from build123d import *

# Parameters (mm, degrees)
SKETCH1_W           = 601
SKETCH1_H           = 1100
SKETCH1_R           = 200
BOSS_EXTRUDE1_DEPTH = 1900
SKETCH2_W           = 1900
SKETCH2_H           = 340
CUT_EXTRUDE1_DEPTH  = 300
SKETCH3_R           = 15
SKETCH3_R_2         = 50
CUT_EXTRUDE2_DEPTH  = 2277.225164609


with BuildPart() as part:
    # Sketch1 → Boss-Extrude1 (new body)
    with BuildSketch(Plane(origin=(0, 0, 0), x_dir=(0, 0, -1), z_dir=(1, 0, 0))):
        with Locations((300.5, 550)):
            Rectangle(SKETCH1_W, SKETCH1_H)
        with Locations(Location((201, 550, 0), (0, 0, 180))):
            Circle(SKETCH1_R, mode=Mode.SUBTRACT)
    extrude(amount=BOSS_EXTRUDE1_DEPTH)

    # Sketch2 → Cut-Extrude1 (cut)
    with BuildSketch(Plane.XY):
        with Locations((950, 550)):
            Rectangle(SKETCH2_W, SKETCH2_H)
    extrude(amount=-CUT_EXTRUDE1_DEPTH, mode=Mode.SUBTRACT)

    # Sketch3 → Cut-Extrude2 (cut, through all)
    with BuildSketch(Plane.XY):
        with Locations((100, 820)):
            Circle(SKETCH3_R)
        with Locations((200, 920)):
            Circle(SKETCH3_R_2)
        with Locations((290, 820)):
            Circle(SKETCH3_R)
        with Locations((480, 820)):
            Circle(SKETCH3_R)
        with Locations((670, 820)):
            Circle(SKETCH3_R)
        with Locations((860, 820)):
            Circle(SKETCH3_R)
        with Locations((1050, 820)):
            Circle(SKETCH3_R)
        with Locations((1240, 820)):
            Circle(SKETCH3_R)
        with Locations((1430, 820)):
            Circle(SKETCH3_R)
        with Locations((1620, 820)):
            Circle(SKETCH3_R)
        with Locations((1810, 820)):
            Circle(SKETCH3_R)
        with Locations((290, 280)):
            Circle(SKETCH3_R)
        with Locations((480, 280)):
            Circle(SKETCH3_R)
        with Locations((670, 280)):
            Circle(SKETCH3_R)
        with Locations((860, 280)):
            Circle(SKETCH3_R)
        with Locations((1050, 280)):
            Circle(SKETCH3_R)
        with Locations((1240, 280)):
            Circle(SKETCH3_R)
        with Locations((1430, 280)):
            Circle(SKETCH3_R)
        with Locations((1620, 280)):
            Circle(SKETCH3_R)
        with Locations((1810, 280)):
            Circle(SKETCH3_R)
        with Locations((100, 280)):
            Circle(SKETCH3_R)
        with Locations((390, 920)):
            Circle(SKETCH3_R_2)
        with Locations((580, 920)):
            Circle(SKETCH3_R_2)
        with Locations((770, 920)):
            Circle(SKETCH3_R_2)
        with Locations((960, 920)):
            Circle(SKETCH3_R_2)
        with Locations((1150, 920)):
            Circle(SKETCH3_R_2)
        with Locations((1340, 920)):
            Circle(SKETCH3_R_2)
        with Locations((1530, 920)):
            Circle(SKETCH3_R_2)
        with Locations((1720, 920)):
            Circle(SKETCH3_R_2)
        with Locations((390, 180)):
            Circle(SKETCH3_R_2)
        with Locations((580, 180)):
            Circle(SKETCH3_R_2)
        with Locations((770, 180)):
            Circle(SKETCH3_R_2)
        with Locations((960, 180)):
            Circle(SKETCH3_R_2)
        with Locations((1150, 180)):
            Circle(SKETCH3_R_2)
        with Locations((1340, 180)):
            Circle(SKETCH3_R_2)
        with Locations((1530, 180)):
            Circle(SKETCH3_R_2)
        with Locations((1720, 180)):
            Circle(SKETCH3_R_2)
        with Locations((200, 180)):
            Circle(SKETCH3_R_2)
    extrude(amount=-CUT_EXTRUDE2_DEPTH, mode=Mode.SUBTRACT)


solid = part.part
Model file for the job. Use its own axes, mm. A direction names the side the tool comes from. Round coordinates to 2 decimals unless told otherwise and drop trailing zeros. Loops run counter-clockwise (first coordinate to the right, second up) from the corner with the lowest first, then second, coordinate; pieces in that order, holes last.
1. Band-saw the part on B-B, the plane z = -201. Count the separate pieces of the cut face and the enclosed holes in it, and give its area (3 significant figures).
Check values:
separate pieces: 2
enclosed holes: 38
area: 1,170,000 mm2
2. Tool access for faces 1 (the cylindrical face through (1366.88, 962.16, -296.29)), 2 (the flat face through (937, 380, -47)): list every direction of +Z, -Z, +X, -X, +Y, -Y with a clear straight run to the whole face (end or side of a thin tool).
Check values:
face 1: +Z, -Z
face 2: +Z, +X, -X
3. Mould opens along X. For faces 3 (the cylindrical face through (1197.69, 195.02, -296.29)), 4 (the cylindrical face through (936.7, 544.05, -400.91)) say: +X half, -X half, draft (parallel to the pull), parting line (faces both ways), or undercut.
Check values:
face 3: undercut
face 4: draft
4. Drop a flat-ended pin along its axis: P1, Ø8, axis at x = 1388.5, y = 735.5, coming from the +Z side. Give the stop position or say it passes through.
Check values:
P1: stops at z = 0
5. Band-saw the part on D-D, the plane x = 187.5. List the corners of the cut face in (y, z), and give its area (3 significant figures).
Check values:
outline: (0, -601) - (131.59, -601) - (131.59, 0) - (0, 0) - close; (228.41, -601) - (871.59, -601) - (871.59, 0) - (720, 0) - (720, -95.64) arc R200 cw (long way) to (380, -95.64) - (380, 0) - (228.41, 0) - close; (968.41, -601) - (1100, -601) - (1100, 0) - (968.41, 0) - close
area: 409,000 mm2
6. Band-saw the part on A-A, the plane x = 1340. List the corners of the cut face in (y, z).
Check values:
outline: (0, -601) - (130, -601) - (130, 0) - (0, 0) - close; (230, -601) - (870, -601) - (870, 0) - (720, 0) - (720, -95.64) arc R200 cw (long way) to (380, -95.64) - (380, 0) - (230, 0) - close; (970, -601) - (1100, -601) - (1100, 0) - (970, 0) - close
7. Wall check: probe 1 along Y at (x, z) = (1390.5, -201); probe 2 along Y at (x, z) = (1530, -443); probe 3 along Y at (x, z) = (803, -556). Give the ranges that are in metal, low to high.
Check values:
probe 1: y = 0 to 350, 750 to 1100
probe 2: y = 0 to 130, 230 to 870, 970 to 1100
probe 3: y = 0 to 142.44, 217.56 to 882.44, 957.56 to 1100
